Could you check a few things on this model? Use its own coordinates, in mm. Round coordinates to 2 decimals unless told otherwise and drop trailing zeros. Write each loop counter-clockwise with the first axis right and the second up, starting at its lowest first coordinate (ties: lowest second). Pieces come first, ordered by that corner, then holes. Notation, with made-up numbers: (-28, 69) -> (9, 69) arc R16 ccw to (9, 81) -> close; hole circle Ø9 at (-7.5, -10). An arc over 180 degrees is marked (long way). One line per question, with ' | ' between items. Start each with the question number.
1. If I drill on line 1 along Y through (x, z) = (-19, 1) (3 decimals); line 2 along Y through (x, z) = (-40.5, 0.5); line 3 along X through (y, z) = (33.5, 2.7), over which ranges is the centre line in solid material (lowest first)? Write a range as [from, to].
2. Imagine slicing it at C-C, the plane x = -33.5. List the corners of the cut face in (y, z) for me (3 decimals).
3. Imagine slicing it at B-B, the plane y = 22. List the corners of the cut face in (x, z) for me, and give its area (3 significant figures).
4. Imagine slicing it at A-A, the plane x = 1. List the corners of the cut face in (y, z) for me (3 decimals), and give its area (3 significant figures).
5. For pin 1 Ø10 at (x, y) = (-53.5, -6) entering from -Z; pin 2 Ø1.8 at (y, z) = (26, 4) entering from +X; pin 3 Ø3.5 at (x, y) = (40, -51.995) entering from +Z; pin 4 Ø3 at (x, z) = (44.5, 4) entering from -Y (3 decimals), each with a flat end and sliding along its axis, tell me the tip position at first contact or that it passes through.
from build123d import *

# Parameters (mm, degrees)
SKETCH1_W           = 170.9
SKETCH1_H           = 115.79
BOSS_EXTRUDE1_DEPTH = 5.9
SKETCH2_W           = 5.9
SKETCH2_H           = 15
SKETCH2_W_2         = 10
SKETCH2_H_2         = 5.9
CUT_EXTRUDE1_DEPTH  = 6.9
CUT_EXTRUDE2_REACH  = 7.9
SKETCH4_W           = 120
SKETCH4_H           = 10
CUT_EXTRUDE3_REACH  = 7.9
SKETCH5_R           = 2.05


with BuildPart() as part:
    # Sketch1 → Boss-Extrude1 (new body)
    with BuildSketch(Plane.XY):
        Rectangle(SKETCH1_W, SKETCH1_H)
    extrude(amount=BOSS_EXTRUDE1_DEPTH)

    # Sketch2 → Cut-Extrude1 (cut, through all)
    with BuildSketch(Plane.XY.offset(5.9)):
        with Locations((-82.5, 25)):
            Rectangle(SKETCH2_W, SKETCH2_H)
        with Locations((-82.5, -25)):
            Rectangle(SKETCH2_W, SKETCH2_H)
        with Locations((82.5, -25)):
            Rectangle(SKETCH2_W, SKETCH2_H)
        with Locations((82.5, 25)):
            Rectangle(SKETCH2_W, SKETCH2_H)
        with Locations((-45, 54.945)):
            Rectangle(SKETCH2_W_2, SKETCH2_H_2)
        with Locations((0, 54.945)):
            Rectangle(SKETCH2_W_2, SKETCH2_H_2)
        with Locations((45, 54.945)):
            Rectangle(SKETCH2_W_2, SKETCH2_H_2)
        with Locations((45, -54.945)):
            Rectangle(SKETCH2_W_2, SKETCH2_H_2)
        with Locations((0, -54.945)):
            Rectangle(SKETCH2_W_2, SKETCH2_H_2)
        with Locations((-45, -54.945)):
            Rectangle(SKETCH2_W_2, SKETCH2_H_2)
    extrude(amount=-CUT_EXTRUDE1_DEPTH, mode=Mode.SUBTRACT)

    # Sketch4 → Cut-Extrude2 (cut, up to next)
    with BuildSketch(Plane.XY.offset(5.9), mode=Mode.PRIVATE) as cut_extrude2_sk1:
        with Locations((0, -30)):
            Rectangle(SKETCH4_W, SKETCH4_H)
    cut_extrude2_tool1 = extrude(cut_extrude2_sk1.sketch, amount=-CUT_EXTRUDE2_REACH, mode=Mode.PRIVATE) & part.part
    add(cut_extrude2_tool1.solids().sort_by_distance((0, -30, 5.9))[0], mode=Mode.SUBTRACT)

    # Sketch5 → Cut-Extrude3 (cut, up to next)
    with BuildSketch(Plane.XY.offset(5.9), mode=Mode.PRIVATE) as cut_extrude3_sk1:
        with Locations((-50, 51.995)):
            Circle(SKETCH5_R)
    cut_extrude3_tool1 = extrude(cut_extrude3_sk1.sketch, amount=-CUT_EXTRUDE3_REACH, mode=Mode.PRIVATE) & part.part
    add(cut_extrude3_tool1.solids().sort_by_distance((-50, 51.995, 5.9))[0], mode=Mode.SUBTRACT)
    # Sketch5 → Cut-Extrude3 (cut, up to next)
    with BuildSketch(Plane.XY.offset(5.9), mode=Mode.PRIVATE) as cut_extrude3_sk2:
        with Locations((-40, 51.995)):
            Circle(SKETCH5_R)
    cut_extrude3_tool2 = extrude(cut_extrude3_sk2.sketch, amount=-CUT_EXTRUDE3_REACH, mode=Mode.PRIVATE) & part.part
    add(cut_extrude3_tool2.solids().sort_by_distance((-40, 51.995, 5.9))[0], mode=Mode.SUBTRACT)
    # Sketch5 → Cut-Extrude3 (cut, up to next)
    with BuildSketch(Plane.XY.offset(5.9), mode=Mode.PRIVATE) as cut_extrude3_sk3:
        with Locations((-5, 51.995)):
            Circle(SKETCH5_R)
    cut_extrude3_tool3 = extrude(cut_extrude3_sk3.sketch, amount=-CUT_EXTRUDE3_REACH, mode=Mode.PRIVATE) & part.part
    add(cut_extrude3_tool3.solids().sort_by_distance((-5, 51.995, 5.9))[0], mode=Mode.SUBTRACT)
    # Sketch5 → Cut-Extrude3 (cut, up to next)
    with BuildSketch(Plane.XY.offset(5.9), mode=Mode.PRIVATE) as cut_extrude3_sk4:
        with Locations((5, 51.995)):
            Circle(SKETCH5_R)
    cut_extrude3_tool4 = extrude(cut_extrude3_sk4.sketch, amount=-CUT_EXTRUDE3_REACH, mode=Mode.PRIVATE) & part.part
    add(cut_extrude3_tool4.solids().sort_by_distance((5, 51.995, 5.9))[0], mode=Mode.SUBTRACT)
    # Sketch5 → Cut-Extrude3 (cut, up to next)
    with BuildSketch(Plane.XY.offset(5.9), mode=Mode.PRIVATE) as cut_extrude3_sk5:
        with Locations((40, 51.995)):
            Circle(SKETCH5_R)
    cut_extrude3_tool5 = extrude(cut_extrude3_sk5.sketch, amount=-CUT_EXTRUDE3_REACH, mode=Mode.PRIVATE) & part.part
    add(cut_extrude3_tool5.solids().sort_by_distance((40, 51.995, 5.9))[0], mode=Mode.SUBTRACT)
    # Sketch5 → Cut-Extrude3 (cut, up to next)
    with BuildSketch(Plane.XY.offset(5.9), mode=Mode.PRIVATE) as cut_extrude3_sk6:
        with Locations((50, 51.995)):
            Circle(SKETCH5_R)
    cut_extrude3_tool6 = extrude(cut_extrude3_sk6.sketch, amount=-CUT_EXTRUDE3_REACH, mode=Mode.PRIVATE) & part.part
    add(cut_extrude3_tool6.solids().sort_by_distance((50, 51.995, 5.9))[0], mode=Mode.SUBTRACT)
    # Sketch5 → Cut-Extrude3 (cut, up to next)
    with BuildSketch(Plane.XY.offset(5.9), mode=Mode.PRIVATE) as cut_extrude3_sk7:
        with Locations((79.55, 32.5)):
            Circle(SKETCH5_R)
    cut_extrude3_tool7 = extrude(cut_extrude3_sk7.sketch, amount=-CUT_EXTRUDE3_REACH, mode=Mode.PRIVATE) & part.part
    add(cut_extrude3_tool7.solids().sort_by_distance((79.55, 32.5, 5.9))[0], mode=Mode.SUBTRACT)
    # Sketch5 → Cut-Extrude3 (cut, up to next)
    with BuildSketch(Plane.XY.offset(5.9), mode=Mode.PRIVATE) as cut_extrude3_sk8:
        with Locations((79.55, 17.5)):
            Circle(SKETCH5_R)
    cut_extrude3_tool8 = extrude(cut_extrude3_sk8.sketch, amount=-CUT_EXTRUDE3_REACH, mode=Mode.PRIVATE) & part.part
    add(cut_extrude3_tool8.solids().sort_by_distance((79.55, 17.5, 5.9))[0], mode=Mode.SUBTRACT)
    # Sketch5 → Cut-Extrude3 (cut, up to next)
    with BuildSketch(Plane.XY.offset(5.9), mode=Mode.PRIVATE) as cut_extrude3_sk9:
        with Locations((79.55, -17.5)):
            Circle(SKETCH5_R)
    cut_extrude3_tool9 = extrude(cut_extrude3_sk9.sketch, amount=-CUT_EXTRUDE3_REACH, mode=Mode.PRIVATE) & part.part
    add(cut_extrude3_tool9.solids().sort_by_distance((79.55, -17.5, 5.9))[0], mode=Mode.SUBTRACT)
    # Sketch5 → Cut-Extrude3 (cut, up to next)
    with BuildSketch(Plane.XY.offset(5.9), mode=Mode.PRIVATE) as cut_extrude3_sk10:
        with Locations((79.55, -32.5)):
            Circle(SKETCH5_R)
    cut_extrude3_tool10 = extrude(cut_extrude3_sk10.sketch, amount=-CUT_EXTRUDE3_REACH, mode=Mode.PRIVATE) & part.part
    add(cut_extrude3_tool10.solids().sort_by_distance((79.55, -32.5, 5.9))[0], mode=Mode.SUBTRACT)
    # Sketch5 → Cut-Extrude3 (cut, up to next)
    with BuildSketch(Plane.XY.offset(5.9), mode=Mode.PRIVATE) as cut_extrude3_sk11:
        with Locations((-40, -51.995)):
            Circle(SKETCH5_R)
    cut_extrude3_tool11 = extrude(cut_extrude3_sk11.sketch, amount=-CUT_EXTRUDE3_REACH, mode=Mode.PRIVATE) & part.part
    add(cut_extrude3_tool11.solids().sort_by_distance((-40, -51.995, 5.9))[0], mode=Mode.SUBTRACT)
    # Sketch5 → Cut-Extrude3 (cut, up to next)
    with BuildSketch(Plane.XY.offset(5.9), mode=Mode.PRIVATE) as cut_extrude3_sk12:
        with Locations((-5, -51.995)):
            Circle(SKETCH5_R)
    cut_extrude3_tool12 = extrude(cut_extrude3_sk12.sketch, amount=-CUT_EXTRUDE3_REACH, mode=Mode.PRIVATE) & part.part
    add(cut_extrude3_tool12.solids().sort_by_distance((-5, -51.995, 5.9))[0], mode=Mode.SUBTRACT)
    # Sketch5 → Cut-Extrude3 (cut, up to next)
    with BuildSketch(Plane.XY.offset(5.9), mode=Mode.PRIVATE) as cut_extrude3_sk13:
        with Locations((5, -51.995)):
            Circle(SKETCH5_R)
    cut_extrude3_tool13 = extrude(cut_extrude3_sk13.sketch, amount=-CUT_EXTRUDE3_REACH, mode=Mode.PRIVATE) & part.part
    add(cut_extrude3_tool13.solids().sort_by_distance((5, -51.995, 5.9))[0], mode=Mode.SUBTRACT)
    # Sketch5 → Cut-Extrude3 (cut, up to next)
    with BuildSketch(Plane.XY.offset(5.9), mode=Mode.PRIVATE) as cut_extrude3_sk14:
        with Locations((40, -51.995)):
            Circle(SKETCH5_R)
    cut_extrude3_tool14 = extrude(cut_extrude3_sk14.sketch, amount=-CUT_EXTRUDE3_REACH, mode=Mode.PRIVATE) & part.part
    add(cut_extrude3_tool14.solids().sort_by_distance((40, -51.995, 5.9))[0], mode=Mode.SUBTRACT)
    # Sketch5 → Cut-Extrude3 (cut, up to next)
    with BuildSketch(Plane.XY.offset(5.9), mode=Mode.PRIVATE) as cut_extrude3_sk15:
        with Locations((50, -51.995)):
            Circle(SKETCH5_R)
    cut_extrude3_tool15 = extrude(cut_extrude3_sk15.sketch, amount=-CUT_EXTRUDE3_REACH, mode=Mode.PRIVATE) & part.part
    add(cut_extrude3_tool15.solids().sort_by_distance((50, -51.995, 5.9))[0], mode=Mode.SUBTRACT)
    # Sketch5 → Cut-Extrude3 (cut, up to next)
    with BuildSketch(Plane.XY.offset(5.9), mode=Mode.PRIVATE) as cut_extrude3_sk16:
        with Locations((-50, -51.995)):
            Circle(SKETCH5_R)
    cut_extrude3_tool16 = extrude(cut_extrude3_sk16.sketch, amount=-CUT_EXTRUDE3_REACH, mode=Mode.PRIVATE) & part.part
    add(cut_extrude3_tool16.solids().sort_by_distance((-50, -51.995, 5.9))[0], mode=Mode.SUBTRACT)
    # Sketch5 → Cut-Extrude3 (cut, up to next)
    with BuildSketch(Plane.XY.offset(5.9), mode=Mode.PRIVATE) as cut_extrude3_sk17:
        with Locations((-79.55, -32.5)):
            Circle(SKETCH5_R)
    cut_extrude3_tool17 = extrude(cut_extrude3_sk17.sketch, amount=-CUT_EXTRUDE3_REACH, mode=Mode.PRIVATE) & part.part
    add(cut_extrude3_tool17.solids().sort_by_distance((-79.55, -32.5, 5.9))[0], mode=Mode.SUBTRACT)
    # Sketch5 → Cut-Extrude3 (cut, up to next)
    with BuildSketch(Plane.XY.offset(5.9), mode=Mode.PRIVATE) as cut_extrude3_sk18:
        with Locations((-79.55, -17.5)):
            Circle(SKETCH5_R)
    cut_extrude3_tool18 = extrude(cut_extrude3_sk18.sketch, amount=-CUT_EXTRUDE3_REACH, mode=Mode.PRIVATE) & part.part
    add(cut_extrude3_tool18.solids().sort_by_distance((-79.55, -17.5, 5.9))[0], mode=Mode.SUBTRACT)
    # Sketch5 → Cut-Extrude3 (cut, up to next)
    with BuildSketch(Plane.XY.offset(5.9), mode=Mode.PRIVATE) as cut_extrude3_sk19:
        with Locations((-79.55, 17.5)):
            Circle(SKETCH5_R)
    cut_extrude3_tool19 = extrude(cut_extrude3_sk19.sketch, amount=-CUT_EXTRUDE3_REACH, mode=Mode.PRIVATE) & part.part
    add(cut_extrude3_tool19.solids().sort_by_distance((-79.55, 17.5, 5.9))[0], mode=Mode.SUBTRACT)
    # Sketch5 → Cut-Extrude3 (cut, up to next)
    with BuildSketch(Plane.XY.offset(5.9), mode=Mode.PRIVATE) as cut_extrude3_sk20:
        with Locations((-79.55, 32.5)):
            Circle(SKETCH5_R)
    cut_extrude3_tool20 = extrude(cut_extrude3_sk20.sketch, amount=-CUT_EXTRUDE3_REACH, mode=Mode.PRIVATE) & part.part
    add(cut_extrude3_tool20.solids().sort_by_distance((-79.55, 32.5, 5.9))[0], mode=Mode.SUBTRACT)


solid = part.part
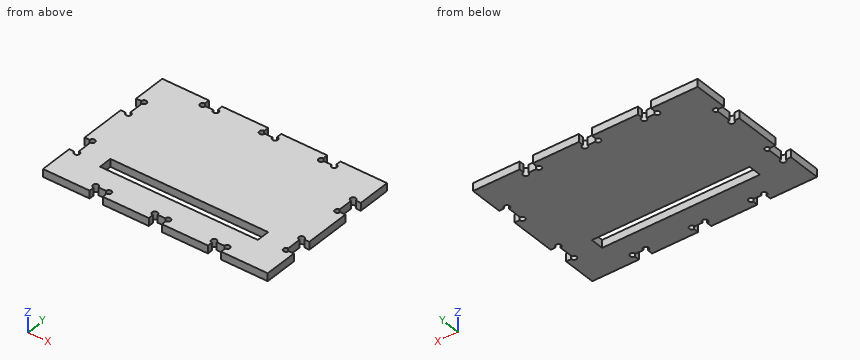
Geometry results:
1) line 1: y = [-57.895, -35], [-25, 57.895] | line 2: y = [-50.01, -35], [-25, 50.01] | line 3: x = [-85.45, -81.34], [-77.76, 77.76], [81.34, 85.45]
2) outline: (-57.895, 0) -> (-35, 0) -> (-35, 5.9) -> (-57.895, 5.9) -> close; (-25, 0) -> (57.895, 0) -> (57.895, 5.9) -> (-25, 5.9) -> close
3) outline: (-79.55, 0) -> (79.55, 0) -> (79.55, 5.9) -> (-79.55, 5.9) -> close | area: 939 mm2
4) outline: (-51.995, 0) -> (-35, 0) -> (-35, 5.9) -> (-51.995, 5.9) -> close; (-25, 0) -> (51.995, 0) -> (51.995, 5.9) -> (-25, 5.9) -> close | area: 555 mm2
5) pin 1: stops at z = 0 | pin 2: stops at x = 79.55 | pin 3: passes through | pin 4: stops at y = -51.995
